Here's how the part is built. I have some questions about the finished solid (model axes, mm). Face numbers are marked on the shaded views. Round coordinates to 2 decimals unless told otherwise and drop trailing zeros. Loops run counter-clockwise (first coordinate to the right, second up) from the corner with the lowest first, then second, coordinate; pieces in that order, holes last. Notation, with made-up numbers: M 83.25,6.5 L 87.25,6.5 A7 cw 87.25,18.5 Z; hole C 43.25,45 d2. An arc over 180 degrees is marked long. Answer as a JSON object with one key per item and string values.
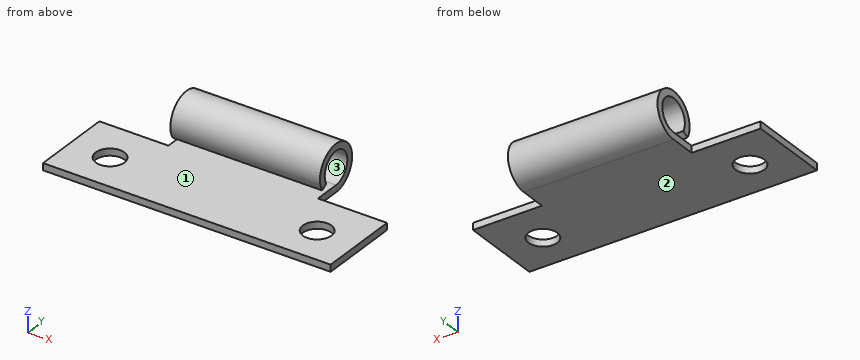
from build123d import *

# Parameters (mm, degrees)
SKETCH_1_W               = 50
SKETCH_1_H               = 18.75
SM_BASE_FLANGE_1_DEPTH   = 1.2
OTHER_START              = -25
OTHER_1_DEPTH            = 50
SKETCH_12_R              = 2.5
CUT_EXTRUDE_3_DEPTH      = 10
CUT_EXTRUDE_1_DEPTH      = 30.203435157
CUT_EXTRUDE_1_DEPTH_BACK = 30.203435157
SKETCH_10_W              = 12
SKETCH_10_H              = 8.6


# Read off the part's stored shape, not the designer's step: 褶边1
# Sheet-metal steps are written as plain solids
with BuildPart() as part:
    # Sketch 1 → 基体-法兰1 (new body)
    with BuildSketch(Plane.XY):
        Rectangle(SKETCH_1_W, SKETCH_1_H)
    extrude(amount=-SM_BASE_FLANGE_1_DEPTH)

    # Other 1 outline → Other 1 (add)
    with BuildSketch(Plane.YZ.offset(OTHER_START)):
        with BuildLine():
            Line((5.867597115, 0.825), (6.906827599, 1.425))
            ThreePointArc((6.906827599, 1.425), (10.8, 5.318172401), (9.375, 0))
            Line((9.375, 0), (9.375, -1.2))
            ThreePointArc((9.375, -1.2), (11.4, 6.357402885), (5.867597115, 0.825))
        make_face()
    extrude(amount=OTHER_1_DEPTH)

    # 草图12 → 切除-拉伸3 (cut)
    with BuildSketch(Plane.XY):
        with Locations((-18, -2.625)):
            Circle(SKETCH_12_R)
        with Locations((18, -2.625)):
            Circle(SKETCH_12_R)
    extrude(amount=-CUT_EXTRUDE_3_DEPTH, mode=Mode.SUBTRACT)

    # 草图10 → 切除-拉伸1 (cut, two sides: drawn at the far end of the back side and taken through both)
    with BuildSketch(Plane.XY.offset(-CUT_EXTRUDE_1_DEPTH_BACK)):
        with Locations((-19, 9.125)):
            Rectangle(SKETCH_10_W, SKETCH_10_H)
        with Locations((19, 9.125)):
            Rectangle(SKETCH_10_W, SKETCH_10_H)
    extrude(amount=CUT_EXTRUDE_1_DEPTH + CUT_EXTRUDE_1_DEPTH_BACK, mode=Mode.SUBTRACT)


solid = part.part
Item 1: Please list where these lines run through material, in increasing order: probe 1 along Y at (x, z) = (18, -0.75) (3 decimals); probe 2 along Y at (x, z) = (-2, 3); probe 3 along Z at (x, y) = (-6, 1). Write a range as from..to.
Resolved:
{"probe 1": "-9.375..-5.125, -0.125..4.825", "probe 2": "5.33..6.53, 12.22..13.42", "probe 3": "-1.2..0"}
Item 2: If we mould it in two halves opening along Z, with no side actions, what happens to the marked faces 1, 2 and 3? For each: pulls with the +Z half, pulls with the -Z half, needs draft (parallel to the pull), parting line crosses it, or undercut.
Resolved:
{"face 1": "undercut", "face 2": "pulls with the -Z half", "face 3": "undercut"}
Item 3: I'm going to push flat-ended pins straight in: pin 1 Ø1.5 at (x, y) = (17, 5) entering from -Z; pin 2 Ø1.3 at (x, z) = (17.5, -0.5) entering from +Y (3 decimals); pin 3 Ø1.5 at (x, y) = (-17, -6) entering from +Z. Where does each tip first touch, or does it pass through?
Resolved:
{"pin 1": "z = -1.2", "pin 2": "y = 4.825", "pin 3": "z = 0"}
Item 4: I want a section at B-B, the plane z = 2.85. Please give me the cut outline in (x, y) (3 decimals), then the cut area to 3 significant figures.
Resolved:
{"outline": "M -13,5.325 L 13,5.325 L 13,6.525 L -13,6.525 Z; M -13,12.225 L 13,12.225 L 13,13.425 L -13,13.425 Z", "area": "62.4 mm²"}
Item 5: I want a section at D-D, the plane x = 10.5. Please give me the cut outline in (y, z) (3 decimals).
Resolved:
{"outline": "M -9.375,-1.2 L 9.375,-1.2 A4.05 ccw long 5.868,0.825 L 6.907,1.425 A2.85 cw long 9.375,0 L -9.375,0 Z"}
Item 6: I want a section at C-C, the plane y = -2. Please give me the cut outline in (x, z), then the cut area to 3 significant figures.
Resolved:
{"outline": "M -25,-1.2 L -20.42,-1.2 L -20.42,0 L -25,0 Z; M -15.58,-1.2 L 15.58,-1.2 L 15.58,0 L -15.58,0 Z; M 20.42,-1.2 L 25,-1.2 L 25,0 L 20.42,0 Z", "area": "48.4 mm²"}
Item 7: I want a section at A-A, the plane x = 18. Please give me the cut outline in (y, z) (3 decimals), then the cut area to 3 significant figures.
Resolved:
{"outline": "M -9.375,-1.2 L -5.125,-1.2 L -5.125,0 L -9.375,0 Z; M -0.125,-1.2 L 4.825,-1.2 L 4.825,0 L -0.125,0 Z", "area": "11.0 mm²"}
